from build123d import *

# Parameters (mm, degrees)
F2_R     = 12.7
F3_DEPTH = 381.001
F5_DEPTH = 381.001


with BuildPart() as f1:
    # F0 (on Top) → F1 (revolve)
    with BuildSketch(Plane.XY):
        with BuildLine():
            Line((-367.592253, 190.5), (-538.48, 190.5))
            Line((-538.48, 190.5), (-538.48, -190.5))
            Line((-538.48, -190.5), (-367.592253, -190.5))
            ThreePointArc((-367.592253, -190.5), (-305.375214, -177.22153), (-254, -139.7))
            Line((-254, -139.7), (-254, 139.7))
            ThreePointArc((-254, 139.7), (-305.375214, 177.22153), (-367.592253, 190.5))
        make_face()
        Polygon((-234.95, 139.7), (-254, 139.7), (-254, -139.7), (-234.95, -139.7), (-234.95, 82.55), (-76.2, 82.55), (-76.2, 101.6), (-204.931125, 101.6), (-234.95, 101.6), (-234.95, 120.65), align=None)
        Polygon((-204.931125, 115.529336), (-234.95, 120.65), (-234.95, 101.6), (-204.931125, 101.6), align=None)
    revolve(axis=Axis((0, 171.656604, 0), (0, 1, 0)))

    # F2 (on face) → F3 (cut, through all)
    with BuildSketch(Plane.XZ.offset(190.5)):
        with Locations((0, 127)):
            Circle(F2_R)
        with Locations((-89.802561, 89.802561)):
            Circle(F2_R)
        with Locations((-127, 0)):
            Circle(F2_R)
        with Locations((-89.802561, -89.802561)):
            Circle(F2_R)
        with Locations((0, -127)):
            Circle(F2_R)
        with Locations((89.802561, -89.802561)):
            Circle(F2_R)
        with Locations((127, 0)):
            Circle(F2_R)
        with Locations((89.802561, 89.802561)):
            Circle(F2_R)
    extrude(amount=-F3_DEPTH, mode=Mode.SUBTRACT)

    # F4 (on face) → F5 (cut, through all)
    with BuildSketch(Plane(origin=(0, 190.5, 0), x_dir=(-1, 0, 0), z_dir=(0, 1, 0))):
        with BuildLine():
            ThreePointArc((29.579128, 537.666984), (0, 538.48), (-29.579128, 537.666984))
            Line((-29.579128, 537.666984), (-19.05, 519.43))
            Line((-19.05, 519.43), (19.05, 519.43))
            Line((19.05, 519.43), (29.579128, 537.666984))
        make_face()
        with BuildLine():
            ThreePointArc((-82.854499, 532.067517), (-111.956287, 526.71292), (-140.720004, 519.767824))
            Line((-140.720004, 519.767824), (-126.629281, 504.118491))
            Line((-126.629281, 504.118491), (-89.361858, 512.039926))
            Line((-89.361858, 512.039926), (-82.854499, 532.067517))
        make_face()
        with BuildLine():
            ThreePointArc((-191.666986, 503.214146), (-219.019548, 491.925958), (-245.710742, 479.152316))
            Line((-245.710742, 479.152316), (-228.674255, 466.774584))
            Line((-228.674255, 466.774584), (-193.868174, 482.27125))
            Line((-193.868174, 482.27125), (-191.666986, 503.214146))
        make_face()
        with BuildLine():
            ThreePointArc((-292.102707, 452.367902), (-316.510603, 435.639471), (-339.962741, 417.595552))
            Line((-339.962741, 417.595552), (-320.725067, 409.030388))
            Line((-320.725067, 409.030388), (-289.90152, 431.425006))
            Line((-289.90152, 431.425006), (-292.102707, 452.367902))
        make_face()
        with BuildLine():
            ThreePointArc((-379.772137, 381.751011), (-400.168626, 360.313449), (-419.356737, 337.787859))
            Line((-419.356737, 337.787859), (-398.758655, 333.409602))
            Line((-398.758655, 333.409602), (-373.264779, 361.72342))
            Line((-373.264779, 361.72342), (-379.772137, 381.751011))
        make_face()
        with BuildLine():
            ThreePointArc((-450.843703, 294.449768), (-466.337359, 269.24), (-480.422831, 243.217216))
            Line((-480.422831, 243.217216), (-459.364575, 243.217216))
            Line((-459.364575, 243.217216), (-440.314575, 276.212784))
            Line((-440.314575, 276.212784), (-450.843703, 294.449768))
        make_face()
        with BuildLine():
            ThreePointArc((-502.211236, 194.279657), (-512.124913, 166.399471), (-520.492142, 138.016813))
            Line((-520.492142, 138.016813), (-499.89406, 142.395071))
            Line((-499.89406, 142.395071), (-488.120513, 178.630324))
            Line((-488.120513, 178.630324), (-502.211236, 194.279657))
        make_face()
        with BuildLine():
            ThreePointArc((-531.629727, 85.618594), (-535.53015, 56.286487), (-537.813449, 26.784414))
            Line((-537.813449, 26.784414), (-518.575775, 35.349578))
            Line((-518.575775, 35.349578), (-514.593241, 73.240862))
            Line((-514.593241, 73.240862), (-531.629727, 85.618594))
        make_face()
        with BuildLine():
            ThreePointArc((-537.813449, -26.784414), (-535.53015, -56.286487), (-531.629727, -85.618594))
            Line((-531.629727, -85.618594), (-514.593241, -73.240862))
            Line((-514.593241, -73.240862), (-518.575775, -35.349578))
            Line((-518.575775, -35.349578), (-537.813449, -26.784414))
        make_face()
        with BuildLine():
            ThreePointArc((-520.492142, -138.016813), (-512.124913, -166.399471), (-502.211236, -194.279657))
            Line((-502.211236, -194.279657), (-488.120513, -178.630324))
            Line((-488.120513, -178.630324), (-499.89406, -142.395071))
            Line((-499.89406, -142.395071), (-520.492142, -138.016813))
        make_face()
        with BuildLine():
            ThreePointArc((-480.422831, -243.217216), (-466.337359, -269.24), (-450.843703, -294.449768))
            Line((-450.843703, -294.449768), (-440.314575, -276.212784))
            Line((-440.314575, -276.212784), (-459.364575, -243.217216))
            Line((-459.364575, -243.217216), (-480.422831, -243.217216))
        make_face()
        with BuildLine():
            ThreePointArc((-419.356737, -337.787859), (-400.168626, -360.313449), (-379.772137, -381.751011))
            Line((-379.772137, -381.751011), (-373.264779, -361.72342))
            Line((-373.264779, -361.72342), (-398.758655, -333.409602))
            Line((-398.758655, -333.409602), (-419.356737, -337.787859))
        make_face()
        with BuildLine():
            ThreePointArc((-339.962741, -417.595552), (-316.510603, -435.639471), (-292.102707, -452.367902))
            Line((-292.102707, -452.367902), (-289.90152, -431.425006))
            Line((-289.90152, -431.425006), (-320.725067, -409.030388))
            Line((-320.725067, -409.030388), (-339.962741, -417.595552))
        make_face()
        with BuildLine():
            ThreePointArc((-245.710742, -479.152316), (-219.019548, -491.925958), (-191.666986, -503.214146))
            Line((-191.666986, -503.214146), (-193.868174, -482.27125))
            Line((-193.868174, -482.27125), (-228.674255, -466.774584))
            Line((-228.674255, -466.774584), (-245.710742, -479.152316))
        make_face()
        with BuildLine():
            ThreePointArc((-140.720004, -519.767824), (-111.956287, -526.71292), (-82.854499, -532.067517))
            Line((-82.854499, -532.067517), (-89.361858, -512.039926))
            Line((-89.361858, -512.039926), (-126.629281, -504.118491))
            Line((-126.629281, -504.118491), (-140.720004, -519.767824))
        make_face()
        with BuildLine():
            ThreePointArc((-29.579128, -537.666984), (0, -538.48), (29.579128, -537.666984))
            Line((29.579128, -537.666984), (19.05, -519.43))
            Line((19.05, -519.43), (-19.05, -519.43))
            Line((-19.05, -519.43), (-29.579128, -537.666984))
        make_face()
        with BuildLine():
            ThreePointArc((82.854499, -532.067517), (111.956287, -526.71292), (140.720004, -519.767824))
            Line((140.720004, -519.767824), (126.629281, -504.118491))
            Line((126.629281, -504.118491), (89.361858, -512.039926))
            Line((89.361858, -512.039926), (82.854499, -532.067517))
        make_face()
        with BuildLine():
            ThreePointArc((191.666986, -503.214146), (219.019548, -491.925958), (245.710742, -479.152316))
            Line((245.710742, -479.152316), (228.674255, -466.774584))
            Line((228.674255, -466.774584), (193.868174, -482.27125))
            Line((193.868174, -482.27125), (191.666986, -503.214146))
        make_face()
        with BuildLine():
            ThreePointArc((292.102707, -452.367902), (316.510603, -435.639471), (339.962741, -417.595552))
            Line((339.962741, -417.595552), (320.725067, -409.030388))
            Line((320.725067, -409.030388), (289.90152, -431.425006))
            Line((289.90152, -431.425006), (292.102707, -452.367902))
        make_face()
        with BuildLine():
            ThreePointArc((379.772137, -381.751011), (400.168626, -360.313449), (419.356737, -337.787859))
            Line((419.356737, -337.787859), (398.758655, -333.409602))
            Line((398.758655, -333.409602), (373.264779, -361.72342))
            Line((373.264779, -361.72342), (379.772137, -381.751011))
        make_face()
        with BuildLine():
            ThreePointArc((450.843703, -294.449768), (466.337359, -269.24), (480.422831, -243.217216))
            Line((480.422831, -243.217216), (459.364575, -243.217216))
            Line((459.364575, -243.217216), (440.314575, -276.212784))
            Line((440.314575, -276.212784), (450.843703, -294.449768))
        make_face()
        with BuildLine():
            ThreePointArc((502.211236, -194.279657), (512.124913, -166.399471), (520.492142, -138.016813))
            Line((520.492142, -138.016813), (499.89406, -142.395071))
            Line((499.89406, -142.395071), (488.120513, -178.630324))
            Line((488.120513, -178.630324), (502.211236, -194.279657))
        make_face()
        with BuildLine():
            ThreePointArc((531.629727, -85.618594), (535.53015, -56.286487), (537.813449, -26.784414))
            Line((537.813449, -26.784414), (518.575775, -35.349578))
            Line((518.575775, -35.349578), (514.593241, -73.240862))
            Line((514.593241, -73.240862), (531.629727, -85.618594))
        make_face()
        with BuildLine():
            ThreePointArc((537.813449, 26.784414), (535.53015, 56.286487), (531.629727, 85.618594))
            Line((531.629727, 85.618594), (514.593241, 73.240862))
            Line((514.593241, 73.240862), (518.575775, 35.349578))
            Line((518.575775, 35.349578), (537.813449, 26.784414))
        make_face()
        with BuildLine():
            ThreePointArc((520.492142, 138.016813), (512.124913, 166.399471), (502.211236, 194.279657))
            Line((502.211236, 194.279657), (488.120513, 178.630324))
            Line((488.120513, 178.630324), (499.89406, 142.395071))
            Line((499.89406, 142.395071), (520.492142, 138.016813))
        make_face()
        with BuildLine():
            ThreePointArc((480.422831, 243.217216), (466.337359, 269.24), (450.843703, 294.449768))
            Line((450.843703, 294.449768), (440.314575, 276.212784))
            Line((440.314575, 276.212784), (459.364575, 243.217216))
            Line((459.364575, 243.217216), (480.422831, 243.217216))
        make_face()
        with BuildLine():
            ThreePointArc((419.356737, 337.787859), (400.168626, 360.313449), (379.772137, 381.751011))
            Line((379.772137, 381.751011), (373.264779, 361.72342))
            Line((373.264779, 361.72342), (398.758655, 333.409602))
            Line((398.758655, 333.409602), (419.356737, 337.787859))
        make_face()
        with BuildLine():
            ThreePointArc((339.962741, 417.595552), (316.510603, 435.639471), (292.102707, 452.367902))
            Line((292.102707, 452.367902), (289.90152, 431.425006))
            Line((289.90152, 431.425006), (320.725067, 409.030388))
            Line((320.725067, 409.030388), (339.962741, 417.595552))
        make_face()
        with BuildLine():
            ThreePointArc((245.710742, 479.152316), (219.019548, 491.925958), (191.666986, 503.214146))
            Line((191.666986, 503.214146), (193.868174, 482.27125))
            Line((193.868174, 482.27125), (228.674255, 466.774584))
            Line((228.674255, 466.774584), (245.710742, 479.152316))
        make_face()
        with BuildLine():
            ThreePointArc((140.720004, 519.767824), (111.956287, 526.71292), (82.854499, 532.067517))
            Line((82.854499, 532.067517), (89.361858, 512.039926))
            Line((89.361858, 512.039926), (126.629281, 504.118491))
            Line((126.629281, 504.118491), (140.720004, 519.767824))
        make_face()
    extrude(amount=-F5_DEPTH, mode=Mode.SUBTRACT)


solid = f1.part
For this review, take the finished solid that the model builds, in its own axes (mm). A direction names the side the tool comes from. Coordinates: 2 decimals unless noted, no trailing zeros. Return JSON: item names as keys, results as strings.
Item 1: Mouldability with a two-part tool opening along X and no side actions: class faces 1 (the flat face through (-225, -139.7, -74)), 2 (the flat face through (-493.925, 2.667, 160.766)), 3 (the flat face through (107.735, 2.667, -508.135)), 4 (the cylindrical face through (268.92, -2.67, 466.52)) as pulls with the +X half, pulls with the -X half, needs draft (parallel to the pull), parting line crosses it, or undercut.
Determined:
{"face 1": "undercut", "face 2": "pulls with the -X half", "face 3": "undercut", "face 4": "pulls with the +X half"}
Item 2: Take a section at A-A (x = 0). State how many separate pieces and enclosed holes the cut face has, then the cut area to 3 significant figures.
Determined:
{"separate pieces": "4", "enclosed holes": "0", "area": "212,000 mm2"}
Item 3: For faces 5 (the cylindrical face through (114.312, 91.942, 0.558)), 6 (the flat face through (211.03, 2.67, -474.63)), 7 (the flat face through (449.706, 2.667, -259.946)), list the 3-axis set-ups (+Z, -Z, +X, -X, +Y, -Y) from which the entire face can be reached by the end or side of a thin tool; tool diameter is ignored.
Determined:
{"face 5": "+Y, -Y", "face 6": "-Z, +Y, -Y", "face 7": "+X, +Y, -Y"}
Item 4: For line 1 (Z direction, x = 0, y = 94); line 2 (Z direction, x = 0, y = 110.5); line 3 (Z direction, x = 441, y = 144.5), list the stretches that pass through material, from the lowest coordinate up.
Determined:
{"line 1": "z = -519.43 to -139.7, -114.3 to -76.2, 76.2 to 114.3, 139.7 to 519.43", "line 2": "z = -519.43 to -204.93, 204.93 to 519.43", "line 3": "z = -309 to -277.4, -275.03 to 275.03, 277.4 to 309"}
Item 5: Insertion check: pin 1 (1 mm diameter, centred on x = 389, y = 122.5, fed in from -Z); pin 2 (17 mm diameter, centred on x = 465.5, y = -41, fed in from +Z); pin 3 (6 mm diameter, centred on y = 93.5, z = 216.5, fed in from +X); pin 4 (20.5 mm diameter, centred on x = 127, z = 0, fed in from +Y). Each pin has a flat end and moves straight along its axis. Give the tip position at first contact, or say it passes through.
Determined:
{"pin 1": "stops at z = -344.8", "pin 2": "stops at z = 247.31", "pin 3": "stops at x = 494.35", "pin 4": "passes through"}
